Autodesk Inventor part; units mm, degrees
ref_plane "YZ Plane" through (0, 0, 0) normal (1, 0, 0) x (0, 1, 0)
ref_plane "XZ Plane" through (0, 0, 0) normal (0, 1, 0) x (-1, 0, 0)
ref_plane "XY Plane" through (0, 0, 0) normal (0, 0, 1) x (1, 0, 0)
sketch "スケッチ1" plane through (0, 0, 0) normal (0, 0, 1) x (1, 0, 0)
  circle A0 centre (0, 0) radius 21.25
  circle A1 centre (0, 0) radius 36.55
  line L0 (0, 0) -> (-28.1908, 10.2606) construction
  line L1 (0, 0) -> (28.1908, 10.2606) construction
  line L2 (-39.5959, 0) -> (43.1917, 0) construction
  line L3 (0, 0) -> (0, 30) construction
  circle A2 centre (-28.1908, 10.2606) radius 2.55
  circle A3 centre (0, 30) radius 2.55
  circle A4 centre (28.1908, 10.2606) radius 2.55
  dimension "d0" = 73.1
  dimension "d1" = 42.5
  dimension "d2" = 30
  dimension "d3" = 30
  dimension "d4" = 20
  dimension "d5" = 20
  dimension "d6" = 30
  dimension "d7" = 5.1
  dimension "d8" = 5.1
  dimension "d9" = 5.1
extrude "押し出し1" add sketch "スケッチ1" along normal blind 10
sketch "スケッチ2" plane through (0, 0, 10) normal (0, 0, 1) x (1, 0, 0)
  line L0 (0, 0) -> (0, -80) construction
  circle A0 centre (0, -80) radius 52.5
  dimension "d12" = 80
  dimension "d16" = 105
extrude "押し出し2" cut sketch "スケッチ2" against normal blind 10
properties part number "円 42.5mm"
Check sheet for the modelled part. Datum: model origin and axes. Units: mm. Give positions to 0.01 mm unless a question says otherwise; leave off trailing zeros. Loops run counter-clockwise (first coordinate to the right, second up) from the corner with the lowest first, then second, coordinate; pieces in that order, holes last. Notation, with made-up numbers: M 23,-9 L 34,-9 A22 ccw 34,7 Z; hole C 34,-28 d10. An arc over 180 degrees is marked long. Return JSON: item names as keys, results as strings. Group by question number.
1. Thickness scan on L1, parallel to Y at x = 0, z = 8.25; L2, parallel to X at y = -19.5, z = 7; L3, parallel to Y at x = 8.5, z = 5.5. Record the ranges inside material, lowest first.
2. Cross-section at B-B on x = 0. Record the boundary of the cut face in (y, z).
3. Cross-section at D-D on z = 4.75. Record the boundary of the cut face in (x, y).
4. Go/stop test with flat-tipped pins: pin 1 (1 mm diameter, centred on x = -26, y = 28.5, fed in from +Z); pin 2 (3 mm diameter, centred on y = -11, z = 6, fed in from -X); pin 3 (2 mm diameter, centred on y = -20.5, z = 7.5, fed in from +X); pin 4 (3 mm diameter, centred on x = -13.5, z = 3.5, fed in from +Y). Record where each tip stops, or that it passes through.
5. Cross-section at A-A on y = 0. Record the boundary of the cut face in (x, z).
6. Mould release check, pull along X, two halves, no side actions. Record for faces 1 (the cylindrical face through (0.3, -27.5, 5.1)), 2 (the cylindrical face through (-1.325, 36.526, 4.93)), 3 (the flat face through (16, 18, 10)): released by +X, released by -X, zero draft, split by the parting line, or undercut.
7. Cross-section at C-C on x = -27.5. Record the boundary of the cut face in (y, z).
Return value:
{
 "1": {"L1": "-27.5 to -21.25, 21.25 to 27.45, 32.55 to 36.55", "L2": "-30.91 to -8.44, 8.44 to 30.91", "L3": "-28.19 to -19.48, 19.48 to 35.55"},
 "2": {"outline": "M -27.5,0 L -21.25,0 L -21.25,10 L -27.5,10 Z; M 21.25,0 L 27.45,0 L 27.45,10 L 21.25,10 Z; M 32.55,0 L 36.55,0 L 36.55,10 L 32.55,10 Z"},
 "3": {"outline": "M -19.16,-31.12 A52.5 cw 19.16,-31.12 A36.55 ccw long Z; hole C -28.19,10.26 d5.1; hole C 0,0 d42.5; hole C 0,30 d5.1; hole C 28.19,10.26 d5.1"},
 "4": {"pin 1": "through", "pin 2": "x = -35.29", "pin 3": "x = 30.91", "pin 4": "y = 34.52"},
 "5": {"outline": "M -36.55,0 L -21.25,0 L -21.25,10 L -36.55,10 Z; M 21.25,0 L 36.55,0 L 36.55,10 L 21.25,10 Z"},
 "6": {"face 1": "undercut", "face 2": "split by the parting line", "face 3": "zero draft"},
 "7": {"outline": "M -24.08,0 L 7.81,0 L 7.81,10 L -24.08,10 Z; M 12.72,0 L 24.08,0 L 24.08,10 L 12.72,10 Z"}
}
